Could you check a few things on this model? Use its own coordinates, in mm. A direction names the side the tool comes from. Give positions to 0.01 mm unless a question says otherwise; leave off trailing zeros. Loops run counter-clockwise (first coordinate to the right, second up) from the corner with the lowest first, then second, coordinate; pieces in that order, holes last. Notation, with made-up numbers: M -27,73.5 L 4,73.5 A29 ccw 4,102.5 Z; hole C 66.25,37.5 d11. An arc over 180 degrees is marked long. Use CSV: the item, a comma, the result in double quotes.
```python
from build123d import *

# Parameters (mm, degrees)
SKETCH_2_W          = 0.406719167
SKETCH_2_H          = 7
CUT_EXTRUDE_1_DEPTH = 5


with BuildPart() as part:
    # 草图1 → 旋转1 (revolve)
    with BuildSketch(Plane.XY):
        Polygon((0, 0), (1.131136209, 0), (1.45, 0.5), (1.45, 31.13125), (1.10625, 31.5), (0.7375, 31.5), (-0.525, 29), (-0.525, 27), (0, 27), align=None)
    revolve(axis=Axis((-1.55, 0, 0), (0, -1, 0)))

    # 草图2 → 切除-拉伸1 (cut, symmetric)
    with BuildSketch(Plane.XY):
        with Locations((-4.428359584, 9.5)):
            Rectangle(SKETCH_2_W, SKETCH_2_H)
        with Locations((1.378359583, 9.5)):
            Rectangle(SKETCH_2_W, SKETCH_2_H)
    extrude(amount=CUT_EXTRUDE_1_DEPTH, both=True, mode=Mode.SUBTRACT)


solid = part.part
```
1. I want a section at C-C, the plane y = 6.5. List the corners of the cut face in (x, z) for me (3 decimals), then the cut area to 3 significant figures.
Outcome:
outline,"M -4.225,-1.358 A3 ccw 1.175,-1.255 L 1.175,1.255 A3 ccw -4.225,1.358 Z; hole C -1.55,0 d3.1"
area,"19.7 mm2"
2. If we mould it in two halves opening along Z, with no side actions, what happens to faces 1 (the face through (-2.916, 29.677, 0.06)), 2 (the face through (-4.547, 16.03, 0.132)), 3 (the face through (1.175, 9, 0))? For each: +Z half, -Z half, draft (parallel to the pull), parting line (faces both ways), or undercut.
Outcome:
face 1,"undercut"
face 2,"parting line"
face 3,"draft"
3. I'm going to push flat-ended pins straight in: pin 1 Ø3 at (x, z) = (-1.55, 0) entering from +Y; pin 2 Ø1.6 at (x, z) = (-2, 0) entering from -Y; pin 3 Ø0.8 at (y, z) = (11, 0.5) entering from +X (3 decimals). Where does each tip first touch, or does it pass through?
Outcome:
pin 1,"y = 29.94"
pin 2,"y = 27"
pin 3,"x = 1.175"
4. I want a section at D-D, the plane y = 28.5. List the corners of the cut face in (x, z) for me (3 decimals).
Outcome:
outline,"C -1.55,0 d6; hole C -1.55,0 d2.05"
5. Please list where these lines run through material, in increasing order: line 1 (Z direction, x = -1.55, y = 17.25); line 2 (Z direction, x = -0.15, y = 29); line 3 (X direction, y = 2, z = -0.35).
Outcome:
line 1,"-3 to -1.55, 1.55 to 3"
line 2,"-2.65 to 2.65"
line 3,"-4.53 to -3.06, -0.04 to 1.43"
6. Which directions (+Z, -Z, +X, -X, +Y, -Y) give clear straight access to the entire face, cutting with the end or side of a thin tool? Please do faces 4 (the face through (-3, 0, -1)), 5 (the face through (-1.886, 13.311, -1.513)), 6 (the face through (-4.225, 9, 0)).
Outcome:
face 4,"+Z, -Z, +X, -X, -Y"
face 5,"-Y"
face 6,"+Z, -Z, -X"
